Here's the drawing with two shaded views (mm, measured from the low corner). I have some questions. Coordinates: 2 decimals unless noted, no trailing zeros. Loops run counter-clockwise (first coordinate to the right, second up) from the corner with the lowest first, then second, coordinate; pieces in that order, holes last. Notation, with made-up numbers: (-22.5, -17.5) - (-6.5, -17.5) arc R35 cw to (-6.5, 14.5) - close; hole circle Ø2 at (86, 66). An arc over 180 degrees is marked (long way). Use a Markdown table: item, result.
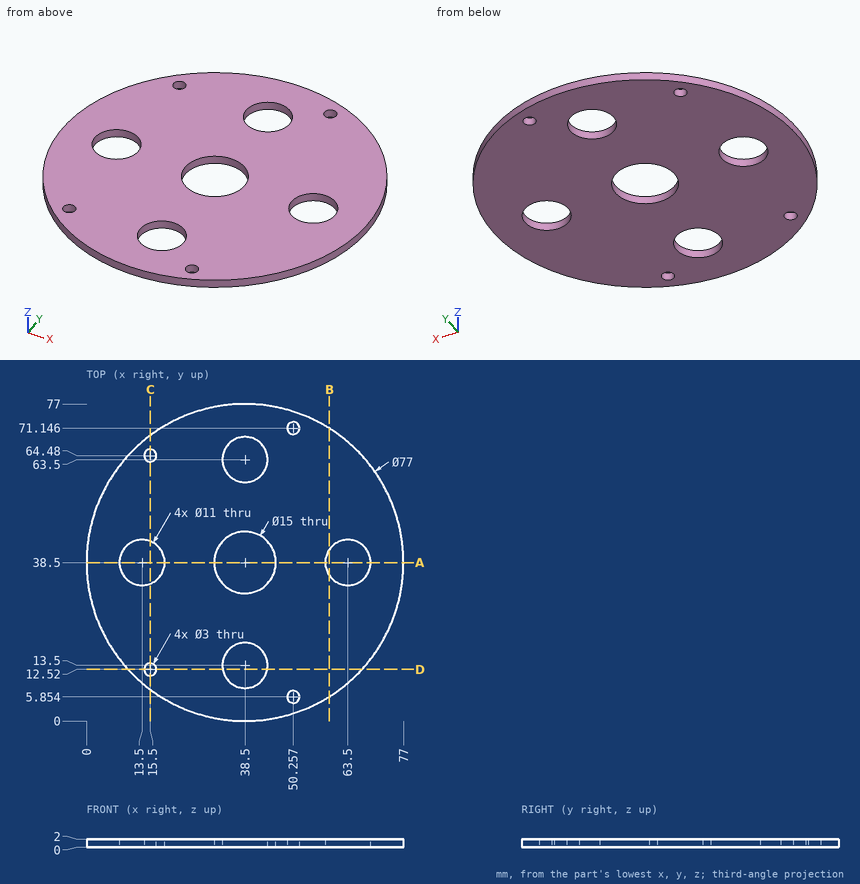
Q1. I want a section at C-C, the plane x = 15.5. Write out the boundary of the cut face in (y, z) (1 decimal), then the cut area to 3 significant figures.
Check values:
| item | result |
|---|---|
| outline | (7.6, 0) - (11, 0) - (11, 2) - (7.6, 2) - close; (14, 0) - (33.4, 0) - (33.4, 2) - (14, 2) - close; (43.6, 0) - (63, 0) - (63, 2) - (43.6, 2) - close; (66, 0) - (69.4, 0) - (69.4, 2) - (66, 2) - close |
| area | 91.0 mm^2 |
Q2. I want a section at B-B, the plane x = 59. Write out the boundary of the cut face in (y, z).
Check values:
| item | result |
|---|---|
| outline | (5.91, 0) - (35.34, 0) - (35.34, 2) - (5.91, 2) - close; (41.66, 0) - (71.09, 0) - (71.09, 2) - (41.66, 2) - close |
Q3. I want a section at D-D, the plane y = 12.52. Write out the boundary of the cut face in (x, z), then the cut area to 3 significant figures.
Check values:
| item | result |
|---|---|
| outline | (10.09, 0) - (14, 0) - (14, 2) - (10.09, 2) - close; (17, 0) - (33.09, 0) - (33.09, 2) - (17, 2) - close; (43.91, 0) - (66.91, 0) - (66.91, 2) - (43.91, 2) - close |
| area | 86.0 mm^2 |
Q4. I want a section at A-A, the plane y = 38.5. Write out the boundary of the cut face in (x, z).
Check values:
| item | result |
|---|---|
| outline | (0, 0) - (8, 0) - (8, 2) - (0, 2) - close; (19, 0) - (31, 0) - (31, 2) - (19, 2) - close; (46, 0) - (58, 0) - (58, 2) - (46, 2) - close; (69, 0) - (77, 0) - (77, 2) - (69, 2) - close |
Q5. Please list where these lines run through material, in increasing order: L1, parallel to Y at x = 37, z = 1.7; L2, parallel to Y at x = 38.5, z = 0.45; L3, parallel to X at y = 43, z = 1.5 (1 decimal). Write a range as from..to.
Check values:
| item | result |
|---|---|
| L1 | 0.03..8.21, 18.79..31.15, 45.85..58.21, 68.79..76.97 |
| L2 | 0..8, 19..31, 46..58, 69..77 |
| L3 | 0.3..10.3, 16.7..32.5, 44.5..60.3, 66.7..76.7 |
